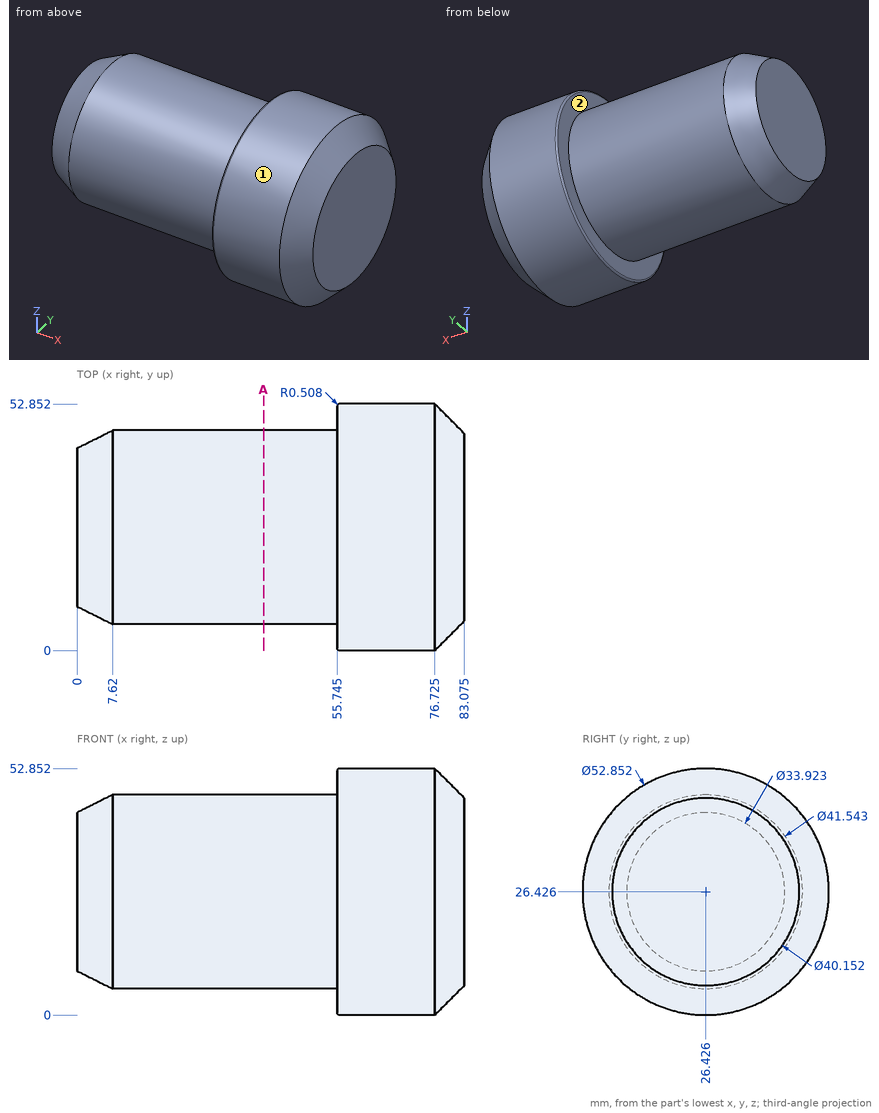
Could you check a few things on this drawing? It's one solid part, dimensions in mm from its lowest x, y, z. A direction names the side the tool comes from. Coordinates: 2 decimals unless noted, no trailing zeros. Write each loop counter-clockwise with the first axis right and the second up, starting at its lowest first coordinate (ties: lowest second). Pieces come first, ordered by that corner, then holes. Notation, with made-up numbers: M 74,80 L 130,80 A25 ccw 130,111 Z; hole C 68.5,-14.5 d7. An arc over 180 degrees is marked long. Answer as CSV lines item,"result". Start each with the question number.
Q1. I need wall thicknesses on probe 1 along Y at (x, z) = (56, 40); probe 2 along Z at (x, y) = (16, 25.5) (1 decimal); probe 3 along X at (y, z) = (34.5, 47.5) (1 decimal). Which ranges of each line are inside material? Lowest first, please. Write a range as [from, to].
Q2. Suppose I cut it at A-A, the plane x = 40. List the corners of the cut face in (y, z) for me, then the cut area to 3 significant figures.
Q3. Will these pins go through, and if not, where does the flat tip stop? pin 1 Ø6 at (x, y) = (74, 42) entering from +Z; pin 2 Ø4 at (x, z) = (14.5, 26) entering from +Y; pin 3 Ø10 at (x, y) = (45.5, 47.5) entering from +Z.
Q4. For the marked faces 1 and 2, which set-ups out of +Z, -Z, +X, -X, +Y, -Y let a thin tool reach every point of the face, with its end or its side?
Entries:
1,probe 1,"y = [3.83, 49.02]"
1,probe 2,"z = [5.7, 47.2]"
1,probe 3,"x = [55.7, 80.6]"
2,outline,"C 26.43,26.43 d41.54"
2,area,"1,360 mm²"
3,pin 1,"stops at z = 49.67"
3,pin 2,"stops at y = 47.2"
3,pin 3,"stops at z = 39.58"
4,face 1,"+X, -X"
4,face 2,"-X"
